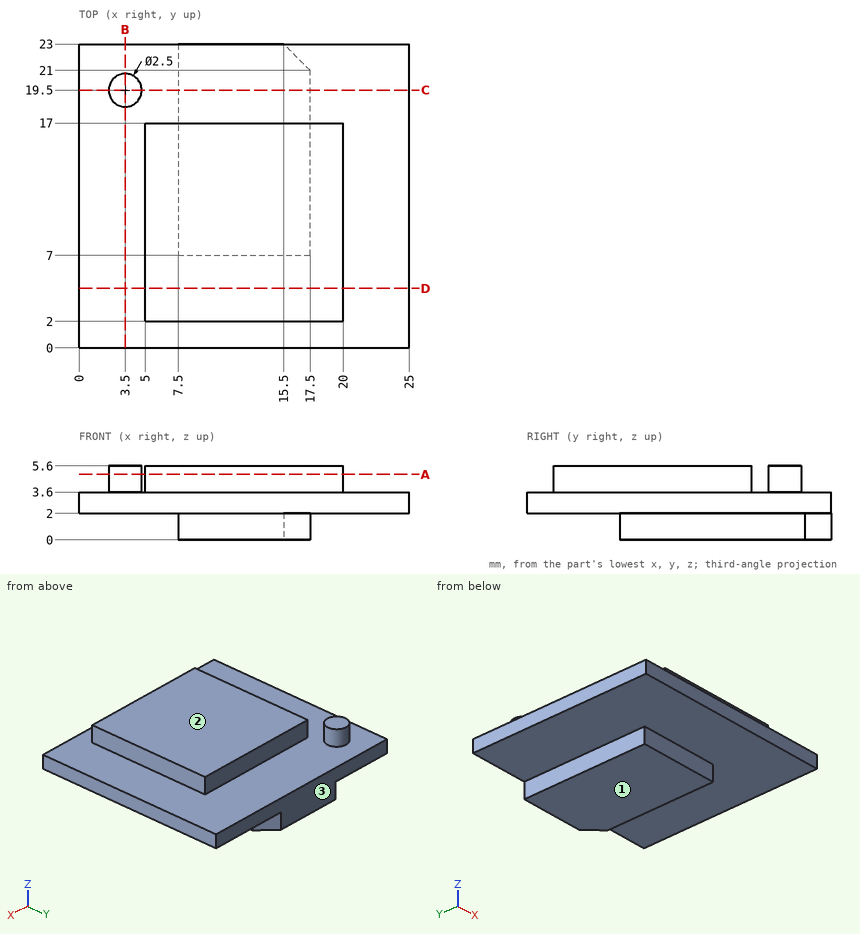
Can you work these out from the drawing? Everything is in mm from the part's minimum corner. Coordinates: 2 decimals unless noted, no trailing zeros. Loops run counter-clockwise (first coordinate to the right, second up) from the corner with the lowest first, then second, coordinate; pieces in that order, holes last. Notation, with made-up numbers: (85, 45) - (117, 45) arc R18 ccw to (117, 79) - close; hole circle Ø2 at (74, 36.5). An arc over 180 degrees is marked (long way). Put each result on its own line as item: value. Start each with the question number.
Item 1: If I drill on line 1 along Z through (x, y) = (4.75, 7); line 2 along Y through (x, z) = (14.5, 1.7); line 3 along Z through (x, y) = (11, 3.75), over which ranges is the centre line in solid material (lowest first)?
Item 2: Suppose I cut it at A-A (z = 4.95). Please give me the cut outline in (x, y), and give its area (3 significant figures).
Item 3: Suppose I cut it at C-C (y = 19.5). Please give me the cut outline in (x, z), and give its area (3 significant figures).
Item 4: Suppose I cut it at D-D (y = 4.5). Please give me the cut outline in (x, z).
Item 5: If we mould it in two halves opening along Z, with no side actions, what happens to the marked faces 1, 2 and 3? For each: +Z half, -Z half, draft (parallel to the pull), parting line (faces both ways), or undercut.
Item 6: For pin 1 (0.6 mm diameter, centred on y = 18.5, z = 0.5, fed in from -X); pin 2 (2 mm diameter, centred on x = 16, z = 4.5, fed in from +Y); pin 3 (0.6 mm diameter, centred on y = 14.5, z = 1, fed in from +X); pin 4 (8 mm diameter, centred on x = 22, y = 8.5, fed in from -Z), each with a flat end and sliding along its axis, tell me the tip position at first contact or that it passes through.
Item 7: Suppose I cut it at B-B (x = 3.5). Please give me the cut outline in (y, z), and give its area (3 significant figures).
Here are the results:
1. line 1: 2 to 3.6
1. line 2: 7 to 23
1. line 3: 2 to 5.6
2. outline: circle Ø2.5 at (3.5, 19.5); (5, 2) - (20, 2) - (20, 17) - (5, 17) - close
2. area: 230 mm²
3. outline: (0, 2) - (7.5, 2) - (7.5, 0) - (17.5, 0) - (17.5, 2) - (25, 2) - (25, 3.6) - (4.75, 3.6) - (4.75, 5.6) - (2.25, 5.6) - (2.25, 3.6) - (0, 3.6) - close
3. area: 65.0 mm²
4. outline: (0, 2) - (25, 2) - (25, 3.6) - (20, 3.6) - (20, 5.6) - (5, 5.6) - (5, 3.6) - (0, 3.6) - close
5. face 1: -Z half
5. face 2: +Z half
5. face 3: draft
6. pin 1: x = 7.5
6. pin 2: y = 23
6. pin 3: x = 17.5
6. pin 4: z = 2
7. outline: (0, 2) - (23, 2) - (23, 3.6) - (20.75, 3.6) - (20.75, 5.6) - (18.25, 5.6) - (18.25, 3.6) - (0, 3.6) - close
7. area: 41.8 mm²
